```python
from build123d import *

# Parameters (mm, degrees)
SKETCH1_W           = 76.2
SKETCH1_H           = 25.4
BOSS_EXTRUDE1_DEPTH = 3.175
SKETCH3_W           = 10.287
SKETCH3_H           = 3.302
SKETCH3_W_2         = 5.334
SKETCH3_W_3         = 3.302
CUT_EXTRUDE1_DEPTH  = 41.286233691


with BuildPart() as part:
    # Sketch1 → Boss-Extrude1 (new body)
    with BuildSketch(Plane(origin=(0, 0, 0), x_dir=(1, 0, 0), z_dir=(0, 1, 0))):
        Rectangle(SKETCH1_W, SKETCH1_H)
    extrude(amount=BOSS_EXTRUDE1_DEPTH)

    # Sketch3 → Cut-Extrude1 (cut, through all)
    with BuildSketch(Plane(origin=(0, 3.175, 0), x_dir=(1, 0, 0), z_dir=(0, 1, 0))):
        with Locations((32.9565, -11.049)):
            Rectangle(SKETCH3_W, SKETCH3_H)
        with Locations((20.32, -11.049)):
            Rectangle(SKETCH3_W_2, SKETCH3_H)
        with Locations((10.16, -11.049)):
            Rectangle(SKETCH3_W_2, SKETCH3_H)
        with Locations((0, -11.049)):
            Rectangle(SKETCH3_W_2, SKETCH3_H)
        with Locations((-10.16, -11.049)):
            Rectangle(SKETCH3_W_2, SKETCH3_H)
        with Locations((-20.32, -11.049)):
            Rectangle(SKETCH3_W_2, SKETCH3_H)
        with Locations((-32.9565, -11.049)):
            Rectangle(SKETCH3_W, SKETCH3_H)
        with Locations((36.449, -4.699)):
            Rectangle(SKETCH3_W_3, SKETCH3_H)
        with Locations((36.449, 1.651)):
            Rectangle(SKETCH3_W_3, SKETCH3_H)
        Polygon((38.1, 6.35), (34.798, 6.35), (34.798, 9.652), (34.798, 12.7), (38.1, 12.7), (38.1, 9.652), align=None)
        Polygon((-34.798, 12.7), (-34.798, 9.652), (-34.798, 6.35), (-38.1, 6.35), (-38.1, 9.652), (-38.1, 12.7), align=None)
        with Locations((-36.449, 1.651)):
            Rectangle(SKETCH3_W_3, SKETCH3_H)
        with Locations((-36.449, -4.699)):
            Rectangle(SKETCH3_W_3, SKETCH3_H)
    extrude(amount=-CUT_EXTRUDE1_DEPTH, mode=Mode.SUBTRACT)


solid = part.part
```
Could you check a few things on this model? Use its own coordinates, in mm. A direction names the side the tool comes from. Coordinates: 2 decimals unless noted, no trailing zeros. Order: outer loops, then holes, each group sorted by start corner. A loop starts at its lowest first (then second) coordinate and runs counter-clockwise, first axis right, second up. Notation, with made-up numbers: M 21,-32.75 L 41,-32.75 A28 ccw 41,-9.75 Z; hole C 76.25,24.5 d2. An arc over 180 degrees is marked long. Use a Markdown table: item, result. Add a question column.
Q1. Which directions (+Z, -Z, +X, -X, +Y, -Y) give clear straight access to the entire face, cutting with the end or side of a thin tool? Please do faces 4 (the flat face through (-34.798, 2, -9)), 5 (the flat face through (34.798, 2, -2)), 6 (the flat face through (36, 2, -6.35)), 7 (the flat face through (17.653, 2, 11)), 8 (the flat face through (-36, 2, 0)).
Q2. I want a section at C-C on x = -22. List the corners of the cut face in (y, z) for me (3 decimals), then the cut area to 3 significant figures.
Q3. I want a section at B-B on z = 4.5. List the corners of the cut face in (x, y) for me (3 decimals).
Q4. If I drill on L1, parallel to X at y = 1.75, z = 11.5; L2, parallel to Z at x = 35, y = 1; L3, parallel to Z at x = -1.5, y = 1.95, over which ranges is the centre line in solid material (lowest first)?
Q5. I want a section at A-A on z = 10.5. List the corners of the cut face in (x, y) for me (3 decimals), then the cut area to 3 significant figures.
Q6. We'd pull the mould along X, two halves only. Please class faces 1 (the flat face through (33, 2, 9.398)), 2 (the flat face through (0, 2, 9.398)), 3 (the flat face through (34.798, 2, -10)): pulls with the +X half, pulls with the -X half, needs draft (parallel to the pull), parting line crosses it, or undercut.
Q7. I'm going to push flat-ended pins straight in: pin 1 (1 mm diameter, centred on x = 36.5, y = 1.5, fed in from -Z); pin 2 (1.5 mm diameter, centred on y = 2, z = -8, fed in from -X); pin 3 (1.6 mm diameter, centred on x = 37, y = 2, fed in from +Z); pin 4 (3 mm diameter, centred on x = 30.5, z = -0.5, fed in from -Y). Where does each tip first touch, or does it pass through?
Checked values:
| question | item | result |
|---|---|---|
| 1 | face 4 | -Z, -X, +Y, -Y |
| 1 | face 5 | +X, +Y, -Y |
| 1 | face 6 | -Z, +X, +Y, -Y |
| 1 | face 7 | +Z, +Y, -Y |
| 1 | face 8 | -X, +Y, -Y |
| 2 | outline | M 0,-12.7 L 3.175,-12.7 L 3.175,9.398 L 0,9.398 Z |
| 2 | area | 70.2 mm² |
| 3 | outline | M -34.798,0 L 34.798,0 L 34.798,3.175 L -34.798,3.175 Z |
| 4 | L1 | -27.81 to -22.99, -17.65 to -12.83, -7.49 to -2.67, 2.67 to 7.49, 12.83 to 17.65, 22.99 to 27.81 |
| 4 | L2 | -6.35 to -3.3, 0 to 3.05, 6.35 to 9.4 |
| 4 | L3 | -12.7 to 9.4 |
| 5 | outline | M -27.813,0 L -22.987,0 L -22.987,3.175 L -27.813,3.175 Z; M -17.653,0 L -12.827,0 L -12.827,3.175 L -17.653,3.175 Z; M -7.493,0 L -2.667,0 L -2.667,3.175 L -7.493,3.175 Z; M 2.667,0 L 7.493,0 L 7.493,3.175 L 2.667,3.175 Z; M 12.827,0 L 17.653,0 L 17.653,3.175 L 12.827,3.175 Z; M 22.987,0 L 27.813,0 L 27.813,3.175 L 22.987,3.175 Z |
| 5 | area | 91.9 mm² |
| 6 | face 1 | needs draft |
| 6 | face 2 | undercut |
| 6 | face 3 | pulls with the +X half |
| 7 | pin 1 | z = -6.35 |
| 7 | pin 2 | x = -34.8 |
| 7 | pin 3 | z = 9.4 |
| 7 | pin 4 | y = 0 |
